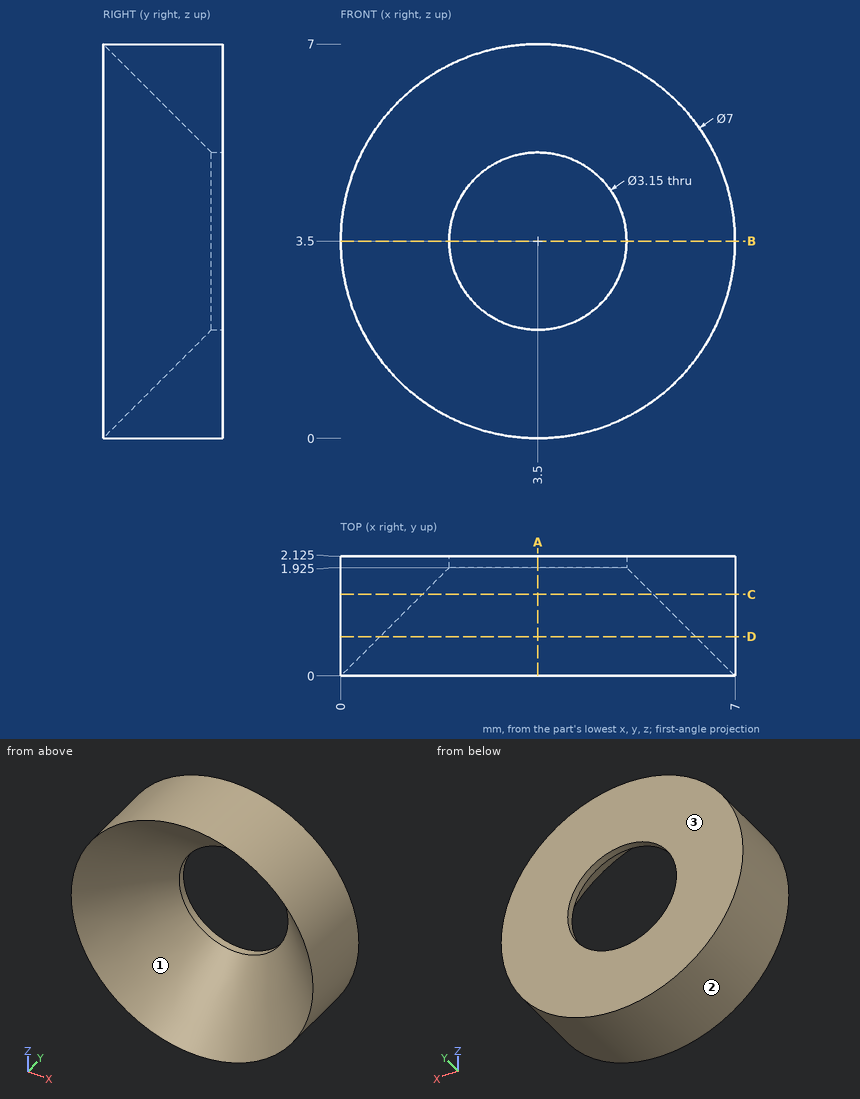
Can you work these out from the drawing? Everything is in mm from the part's minimum corner. Coordinates: 2 decimals unless noted, no trailing zeros. Loops run counter-clockwise (first coordinate to the right, second up) from the corner with the lowest first, then second, coordinate; pieces in that order, holes last.
1. Imagine slicing it at C-C, the plane y = 1.45. Please give me the cut outline in (x, z), and give its area (3 significant figures).
2. Imagine slicing it at D-D, the plane y = 0.7. Please give me the cut outline in (x, z).
3. If we mould it in two halves opening along Z, with no side actions, what happens to the marked faces 1, 2 and 3? For each: pulls with the +Z half, pulls with the -Z half, needs draft (parallel to the pull), parting line crosses it, or undercut.
4. For P1, Ø3, axis at x = 3.5, z = 3.5, coming from the -Y side; P2, Ø1, axis at x = 2.5, z = 5, coming from the -Y side; P3, Ø1, axis at y = 0.5, z = 1.5, coming from the +X side, each with a flat end and sliding along its axis, tell me the tip position at first contact or that it passes through.
5. Imagine slicing it at B-B, the plane z = 3.5. Please give me the cut outline in (x, y) (3 decimals), and give its area (3 significant figures).
6. I need wall thicknesses on L1, parallel to Z at x = 3.5, y = 2.05 (3 decimals); L2, parallel to Z at x = 4.5, y = 0.9. Which ranges of each line are inside material? Lowest first, please.
7. Imagine slicing it at A-A, the plane x = 3.5. Please give me the cut outline in (y, z) (3 decimals), and give its area (3 significant figures).
Taken from the geometry:
1. outline: circle Ø7 at (3.5, 3.5); hole circle Ø4.1 at (3.5, 3.5)
1. area: 25.3 mm2
2. outline: circle Ø7 at (3.5, 3.5); hole circle Ø5.6 at (3.5, 3.5)
3. face 1: undercut
3. face 2: parting line crosses it
3. face 3: needs draft
4. P1: passes through
4. P2: stops at y = 1.2
4. P3: stops at x = 6.66
5. outline: (0, 0) - (1.925, 1.925) - (1.925, 2.125) - (0, 2.125) - close; (5.075, 1.925) - (7, 0) - (7, 2.125) - (5.075, 2.125) - close
5. area: 4.48 mm2
6. L1: z = 0 to 1.925, 5.075 to 7
6. L2: z = 0.15 to 1.1, 5.9 to 6.85
7. outline: (0, 0) - (2.125, 0) - (2.125, 1.925) - (1.925, 1.925) - close; (0, 7) - (1.925, 5.075) - (2.125, 5.075) - (2.125, 7) - close
7. area: 4.48 mm2
